Here's how the part is built. I have some questions about the finished solid (model axes, mm). Face numbers are marked on the shaded views. A direction names the side the tool comes from. Round coordinates to 2 decimals unless told otherwise and drop trailing zeros. Order: outer loops, then holes, each group sorted by start corner. A loop starts at its lowest first (then second) coordinate and runs counter-clockwise, first axis right, second up. Notation, with made-up numbers: M -34.5,-25 L -6.5,-25 A35 cw -6.5,14 Z; hole C 86,49 d11. An arc over 180 degrees is marked long. Answer as CSV lines item,"result". Start each with the question number.
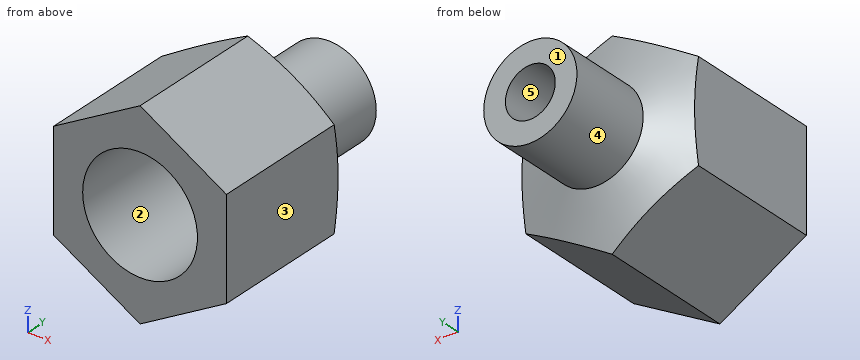
Autodesk Inventor part; units mm, degrees
ref_plane "Work Plane1" through (0, 26.8224, 0) normal (0, -1, 0) x (1, 0, 0)
ref_plane "YZ Plane" through (0, 0, 0) normal (1, 0, 0) x (0, 1, 0)
ref_plane "XZ Plane" through (0, 0, 0) normal (0, 1, 0) x (-1, 0, 0)
sketch "Sketch1" plane through (0, 0, 0) normal (0, 1, 0) x (-1, 0, 0)
  circle A0 centre (0, 0) radius 9.5504 construction
  line L0 (9.5504, -5.5139) -> (0, -11.0279)
  line L1 (0, -11.0279) -> (-9.5504, -5.5139)
  line L2 (-9.5504, -5.5139) -> (-9.5504, 5.5139)
  line L3 (-9.5504, 5.5139) -> (0, 11.0279)
  line L4 (0, 11.0279) -> (9.5504, 5.5139)
  line L5 (9.5504, 5.5139) -> (9.5504, -5.5139)
  circle A1 centre (0, 0) radius 6.35
  point P0 (9.5504, 0)
  dimension "d0" = 19.1008
  dimension "d1" = 12.7
extrude "Extrusion1" add sketch "Sketch1" along normal blind 15.24
ref_plane "Work Plane1" through (0, 26.8224, 0) normal (0, -1, 0) x (1, 0, 0)
sketch "Sketch2" plane through (0, 26.8224, 0) normal (0, -1, 0) x (1, 0, 0)
  circle A0 centre (0, 0) radius 2.7559
  circle A1 centre (0, 0) radius 5.1562
  dimension "d5" = 5.5118
  dimension "d6" = 10.3124
extrude "Extrusion2" add sketch "Sketch2" along normal blind 9.3726
sketch "Sketch3" plane through (0, 0, 0) normal (1, 0, 0) x (0, 1, 0)
  line L0 (15.24, -11.0279) -> (0, -11.0279) construction
  line L1 (0, -11.0279) -> (0, -6.35) construction
  line L2 (0, -6.35) -> (15.24, -6.35) construction
  line L3 (15.24, -6.35) -> (15.24, -11.0279) construction
  line L4 (0, 11.0279) -> (15.24, 11.0279) construction
  line L5 (15.24, 11.0279) -> (15.24, 6.35) construction
  line L6 (15.24, 6.35) -> (0, 6.35) construction
  line L7 (0, 6.35) -> (0, 11.0279) construction
  line L8 (26.8224, -5.1562) -> (17.4498, -5.1562) construction
  line L9 (17.4498, -5.1562) -> (17.4498, -2.7559) construction
  line L10 (17.4498, -2.7559) -> (26.8224, -2.7559) construction
  line L11 (26.8224, -2.7559) -> (26.8224, -5.1562) construction
  line L12 (17.4498, 5.1562) -> (26.8224, 5.1562) construction
  line L13 (26.8224, 5.1562) -> (26.8224, 2.7559) construction
  line L14 (26.8224, 2.7559) -> (17.4498, 2.7559) construction
  line L15 (17.4498, 2.7559) -> (17.4498, 5.1562) construction
  line L16 (17.4498, 5.1562) -> (17.4498, -5.1562)
  line L17 (17.4498, -2.7559) -> (17.4498, -5.1562)
  line L18 (17.4498, -5.1562) -> (15.24, -11.0279)
  line L19 (15.24, -6.35) -> (17.4498, -2.7559)
  line L20 (0, 0) -> (26.8224, 0) construction
  line L21 (15.24, -6.35) -> (15.24, -11.0279)
revolve "Revolution1" add sketch "Sketch3" angle 360 about axis through (0, 0, 0) along (0, 1, 0)
sketch "Sketch4" plane through (0, 0, 0) normal (0, -1, 0) x (1, 0, 0)
  circle A0 centre (0, 0) radius 6.35 construction
  line L0 (9.5504, -5.5139) -> (0, -11.0279)
  line L1 (0, -11.0279) -> (-9.5504, -5.5139)
  line L2 (-9.5504, -5.5139) -> (-9.5504, 5.5139)
  line L3 (-9.5504, 5.5139) -> (0, 11.0279)
  line L4 (0, 11.0279) -> (9.5504, 5.5139)
  line L5 (9.5504, 5.5139) -> (9.5504, -5.5139)
  line L6 (9.5504, 5.5139) -> (0, 11.0279)
  circle A1 centre (0, 0) radius 11.0279
extrude "Extrusion3" cut sketch "Sketch4" against normal through all contours A1 L0 | L5 A1 | A1 L1 | L4 A1 | A1 L2 | L3 A1
properties part number "am-2381" material "Brass"
Item 1: If we section it at C-C on y = 18.5: Please give me the cut outline in (x, z).
Item 2: If I drill on line 1 along Z through (x, y) = (0, 19.5); line 2 along X through (y, z) = (3.5, 0), over which ranges is the centre line in solid material (lowest first)?
Item 3: We'd pull the mould along Z, two halves only. Please class the marked faces 3, 4 and 5: pulls with the +Z half, pulls with the -Z half, needs draft (parallel to the pull), parting line crosses it, or undercut.
Item 4: Which directions (+Z, -Z, +X, -X, +Y, -Y) give clear straight access to the entire face, cutting with the end or side of a thin tool? Please do the marked faces 1 and 2.
Item 5: If we section it at A-A on z = 0: Please give me the cut outline in (x, y), and give its area (3 significant figures).
Item 6: For P1, Ø10, axis at y = 24, z = 6.5, coming from the +X side; P2, Ø8, axis at y = 23, z = 4, coming from the +X side; P3, Ø4, axis at x = -5.5, y = 16, coming from the -Z side, each with a flat end and sliding along its axis, tell me the tip position at first contact or that it passes through.
Item 7: If we section it at B-B on y = 13.5: Please give me the cut outline in (x, z).
Geometry says:
1,outline,"C 0,0 d10.31; hole C 0,0 d5.51"
2,line 1,"-5.16 to -2.76, 2.76 to 5.16"
2,line 2,"-9.55 to -6.35, 6.35 to 9.55"
3,face 3,"needs draft"
3,face 4,"parting line crosses it"
3,face 5,"undercut"
4,face 1,"+Z, -Z, +X, -X, +Y"
4,face 2,"-Y"
5,outline,"M -9.55,0 L -6.35,0 L -6.35,15.24 L -2.76,17.45 L -2.76,26.82 L -5.16,26.82 L -5.16,17.45 L -9.55,15.8 Z; M 2.76,17.45 L 6.35,15.24 L 6.35,0 L 9.55,0 L 9.55,15.8 L 5.16,17.45 L 5.16,26.82 L 2.76,26.82 Z"
5,area,"157 mm²"
6,P1,"x = 4.93"
6,P2,"x = 5.16"
6,P3,"z = -9"
7,outline,"M -9.55,-5.51 L 0,-11.03 L 9.55,-5.51 L 9.55,5.51 L 0,11.03 L -9.55,5.51 Z; hole C 0,0 d12.7"
